For this review, take the finished solid that the model builds, in its own axes (mm). Face numbers are marked on the shaded views. A direction names the side the tool comes from. Give positions to 0.01 mm unless a question says otherwise; leave off trailing zeros. Order: outer loops, then holes, each group sorted by start corner. A loop starts at its lowest first (then second) coordinate and runs counter-clockwise, first axis right, second up. Notation, with made-up numbers: (37.5, -6.75) -> (62.5, -6.75) arc R18 cw to (62.5, 4.25) -> close; hole circle Ø10 at (4, 21.5). An arc over 180 degrees is marked (long way). Use CSV: the item, a comma, the result in double quotes. Start each with the question number.
Autodesk Inventor part; units mm, degrees
ref_plane "YZ Plane" through (0, 0, 0) normal (1, 0, 0) x (0, 1, 0)
ref_plane "XZ Plane" through (0, 0, 0) normal (0, 1, 0) x (-1, 0, 0)
ref_plane "XY Plane" through (0, 0, 0) normal (0, 0, 1) x (1, 0, 0)
sketch "스케치1" plane through (0, 0, 0) normal (0, 1, 0) x (-1, 0, 0)
  line L0 (4.1347, 105.7038) -> (-100.8653, 105.7038)
  line L1 (-100.8653, 105.7038) -> (-100.8653, -184.2962)
  line L2 (-100.8653, -184.2962) -> (4.1347, -184.2962)
  line L3 (4.1347, -184.2962) -> (4.1347, 105.7038)
  point P0 (0, 0)
  dimension "d0" = 105
  dimension "d1" = 290
sketch "스케치2" plane through (0, 0, 0) normal (0, 1, 0) x (-1, 0, 0)
  point P0 (0, 0)
sketch "스케치3" plane through (0, 0, 0) normal (0, 1, 0) x (-1, 0, 0)
  point P0 (0, 0)
sketch "스케치4" plane through (0, 0, 0) normal (0, 1, 0) x (-1, 0, 0)
  point P0 (0, 0)
extrude "돌출1" add sketch "스케치1" along normal blind 100
sketch "스케치5" plane through (100.8653, 0, 105.7038) normal (1, 0, 0) x (0, 0, -1)
  line L0 (0, 0) -> (290, 0)
  line L1 (290, 0) -> (285, 0)
  line L2 (285, 0) -> (285, 5)
  line L3 (285, 5) -> (290, 5)
  line L4 (290, 5) -> (290, 0)
  line L5 (290, 0) -> (290, 100)
  line L6 (290, 100) -> (285, 100)
  line L7 (285, 100) -> (285, 95)
  line L8 (285, 95) -> (290, 95)
  line L9 (290, 95) -> (290, 100)
  line L10 (285, 5) -> (35, 5)
  line L11 (35, 5) -> (35, 95)
  line L12 (35, 95) -> (285, 95)
  line L13 (285, 95) -> (285, 5)
  point P0 (105.7038, 0)
  dimension "d4" = 5
  dimension "d5" = 5
  dimension "d6" = 5
  dimension "d7" = 5
  dimension "d8" = 250
  dimension "d9" = 90
extrude "돌출2" cut sketch "스케치5" against normal blind 100 contours L10 L11 L12 L13
sketch "스케치6" plane through (100.8653, 0, 105.7038) normal (1, 0, 0) x (0, 0, -1)
  point P0 (105.7038, 0)
sketch "스케치7" plane through (100.8653, 0, 105.7038) normal (1, 0, 0) x (0, 0, -1)
  line L0 (285, 5) -> (35, 5)
  line L1 (35, 5) -> (11, 5)
  line L2 (11, 5) -> (11, 95)
  line L3 (11, 95) -> (35, 95)
  line L4 (35, 95) -> (35, 5)
  point P0 (105.7038, 0)
  dimension "d12" = 24
extrude "돌출3" cut sketch "스케치7" against normal blind 100
sketch "스케치8" plane through (-4.1347, 0, 105.7038) normal (0, 0, 1) x (1, 0, 0)
  circle A0 centre (22.6105, 17.0226) radius 10.2543
  point P0 (4.1347, 0)
sketch "스케치11" plane through (-4.1347, 0, -184.2962) normal (-1, 0, 0) x (0, 0, 1)
  point P0 (184.2962, 0)
sketch "스케치9" plane through (-4.1347, 0, -184.2962) normal (-1, 0, 0) x (0, 0, 1)
  line L0 (290, 100) -> (0, 100)
  line L1 (0, 100) -> (5, 100)
  line L2 (5, 100) -> (5, 95)
  line L3 (5, 95) -> (0, 95)
  line L4 (0, 95) -> (0, 100)
  line L5 (0, 0) -> (5, 0)
  line L6 (0, 0) -> (290, 0)
  line L7 (5, 0) -> (75, 0)
  line L8 (5, 0) -> (75, 0) construction
  line L9 (75, 0) -> (140, 0)
  line L10 (75, 0) -> (184.2962, 0)
  dimension "d15" = 5
  dimension "d16" = 5
  dimension "d17" = 5
  dimension "d18" = 70
  dimension "d19" = 0
  dimension "d20" = 65
sketch "스케치12" plane through (-4.1347, 0, -184.2962) normal (-1, 0, 0) x (0, 0, 1)
  point P0 (184.2962, 0)
sketch "스케치10" plane through (0, 0, 0) normal (0, -1, 0) x (1, 0, 0)
  point P0 (0, 0)
sketch "스케치13" plane through (-4.1347, 0, -184.2962) normal (-1, 0, 0) x (0, 0, 1)
  point P0 (184.2962, 0)
sketch "스케치14" plane through (0, 0, 0) normal (0, -1, 0) x (1, 0, 0)
  line L0 (-4.1347, -184.2962) -> (-4.1347, 105.7038)
  line L1 (-4.1347, -110.8863) -> (100.8653, -110.8863)
  line L2 (100.8653, 105.7038) -> (100.8653, -184.2962)
  line L3 (100.8653, -110.8863) -> (40.8653, -110.8863)
  line L4 (40.8653, -110.8863) -> (40.8653, -50.8863)
  line L5 (40.8653, -50.8863) -> (100.8653, -50.8863)
  line L6 (100.8653, -50.8863) -> (100.8653, -110.8863)
  point P0 (0, 0)
  dimension "d21" = 60
  dimension "d22" = 60
extrude "돌출4" cut sketch "스케치14" against normal blind 80
sketch "스케치15" plane through (0, 0, 0) normal (0, -1, 0) x (1, 0, 0)
  line L0 (100.8653, -184.2962) -> (-4.1347, -184.2962)
  line L1 (100.8653, -184.2962) -> (100.8653, -169.2962)
  line L2 (100.8653, -110.8863) -> (100.8653, -184.2962)
  line L3 (100.8653, -169.2962) -> (100.8653, -131.7962)
  circle A0 centre (100.8653, -131.7962) radius 37.5
  point P0 (0, 0)
  dimension "d25" = 15
  dimension "d26" = 37.5
  dimension "d27" = 75
extrude "돌출5" cut sketch "스케치15" against normal blind 80
sketch "스케치16" plane through (0, 0, 0) normal (0, -1, 0) x (1, 0, 0)
  arc A0 (69.7361, -110.8863) -> (100.8653, -169.2962) centre (100.8653, -131.7962) ccw
  line L0 (100.8653, -169.2962) -> (100.8653, -94.2962)
  line L1 (100.8653, 94.7038) -> (100.8653, -179.2962)
  line L2 (100.8653, -169.2962) -> (175.8653, -169.2962) construction
  line L3 (100.8653, -94.2962) -> (100.8653, -34.2962)
  line L4 (100.8653, -34.2962) -> (100.8653, 3.2038)
  circle A1 centre (100.8653, 3.2038) radius 37.5
  point P0 (0, 0)
  point P1 (100.8653, 40.7038)
  dimension "d30" = 75
  dimension "d31" = 90
  dimension "d32" = 60
  dimension "d33" = 37.5
  dimension "d34" = 180
  dimension "d35" = 75
extrude "돌출6" cut sketch "스케치16" against normal blind 8300 contours L1 A1 picked at (87.6481, -17.8312)
sketch "스케치17" plane through (0, 0, 0) normal (0, -1, 0) x (1, 0, 0)
  line L0 (100.8653, -34.2962) -> (100.8653, -184.2962)
  line L1 (100.8653, -184.2962) -> (100.8653, -169.0212)
  line L2 (100.8653, -169.0212) -> (100.8653, -131.5212)
  circle A0 centre (100.8653, -131.5212) radius 37.5
  point P0 (0, 0)
  point P1 (100.8653, -94.0212)
  dimension "d38" = 15.275
  dimension "d39" = 37.5
  dimension "d40" = 75
extrude "돌출7" cut sketch "스케치17" against normal blind 8300 contours L0 A0 picked at (87.6481, -152.5562)
sketch "스케치18" plane through (-4.1347, 0, -184.2962) normal (-1, 0, 0) x (0, 0, 1)
  line L0 (0, 0) -> (0, 100)
  line L1 (0, 50) -> (260, 50)
  line L2 (0, 50) -> (260, 50) construction
  point P0 (184.2962, 0)
  dimension "d43" = 260
  dimension "d44" = 0
sketch "스케치19" plane through (-4.1347, 0, -184.2962) normal (-1, 0, 0) x (0, 0, 1)
  line L0 (259.9404, 50.2138) -> (259.9404, 99.3471)
  line L1 (259.9404, 99.3471) -> (259.9404, 100)
  line L2 (290, 100) -> (225, 100)
  line L3 (290, 0) -> (225, 0)
  line L4 (259.9404, 100) -> (290, 100)
  line L5 (290, 100) -> (290, 0)
  line L6 (290, 0) -> (259.9404, 0)
  line L7 (259.9404, 0) -> (259.9404, 100)
  point P0 (184.2962, 0)
extrude "돌출8" cut sketch "스케치19" against normal blind 50
sketch "스케치24" plane through (100.8653, 0, -184.2962) normal (0, 0, -1) x (-1, 0, 0)
  line L0 (0, 0) -> (0, 5)
  line L1 (103, 100) -> (0, 100)
  line L2 (0, 100) -> (0, 0)
  line L3 (0, 0) -> (103, 0)
  line L4 (103, 0) -> (103, 100)
  point P0 (100.8653, 0)
extrude "돌출12" cut sketch "스케치24" against normal blind 3
sketch "스케치26" plane through (100.8653, 0, 105.7038) normal (0, 0, 1) x (1, 0, 0)
  line L0 (-55, 100) -> (0, 100)
  line L1 (0, 5) -> (0, 0)
  line L2 (-55, 100) -> (0, 100)
  line L3 (0, 100) -> (0, 0)
  line L4 (0, 0) -> (-55, 0)
  line L5 (-55, 0) -> (-55, 100)
  point P0 (-100.8653, 0)
extrude "돌출14" cut sketch "스케치26" against normal blind 7
fillet "모깎기7" radius 2 14 edges at (45.8653, 50, 98.7038) (73.3653, 100, 98.7038) (73.3653, 0, 98.7038) (45.8653, 50, 94.7038) (45.8653, 5, 85.1739) (23.3653, 5, 75.6441) (0.8653, 50, 75.6441) (-4.1347, 50, 75.6441) (23.3653, 95, 75.6441) (20.8653, 100, 75.6441) (20.8653, 0, 75.6441) (45.8653, 95, 85.1739) (45.8653, 100, 87.1739) (45.8653, 0, 87.1739)
sketch "스케치20" plane through (-4.1347, 98, -184.2962) normal (-1, 0, 0) x (0, 0, 1)
  line L0 (99.3624, -73.1284) -> (157.5725, -73.1284)
  line L1 (157.5725, -73.1284) -> (157.5725, -19.1517)
  line L2 (157.5725, -19.1517) -> (99.3624, -19.1517)
  line L3 (99.3624, -19.1517) -> (99.3624, -73.1284)
  point P0 (184.2962, -98)
sketch "스케치21" plane through (-14.1347, 98, -184.2962) normal (-1, 0, 0) x (0, 0, 1)
  line L0 (87.1912, -87.9455) -> (166.5686, -87.9455)
  line L1 (166.5686, -87.9455) -> (166.5686, -6.4514)
  line L2 (166.5686, -6.4514) -> (87.1912, -6.4514)
  line L3 (87.1912, -6.4514) -> (87.1912, -87.9455)
  line L4 (87.1912, -87.9455) -> (166.5686, -6.4514) construction
  line L5 (166.5686, -87.9455) -> (87.1912, -6.4514) construction
  point P0 (184.2962, -98)
  point P1 (126.8799, -47.1984)
sketch "스케치22" plane through (-24.1347, 98, -184.2962) normal (-1, 0, 0) x (0, 0, 1)
  line L0 (162.3351, -80.537) -> (95.6581, -80.537)
  line L1 (95.6581, -80.537) -> (95.6581, -12.8016)
  line L2 (95.6581, -12.8016) -> (162.3351, -12.8016)
  line L3 (162.3351, -12.8016) -> (162.3351, -80.537)
  line L4 (162.3351, -80.537) -> (95.6581, -12.8016) construction
  line L5 (95.6581, -80.537) -> (162.3351, -12.8016) construction
  point P0 (184.2962, -98)
  point P1 (128.9966, -46.6693)
properties part number "차체 뚜껑"
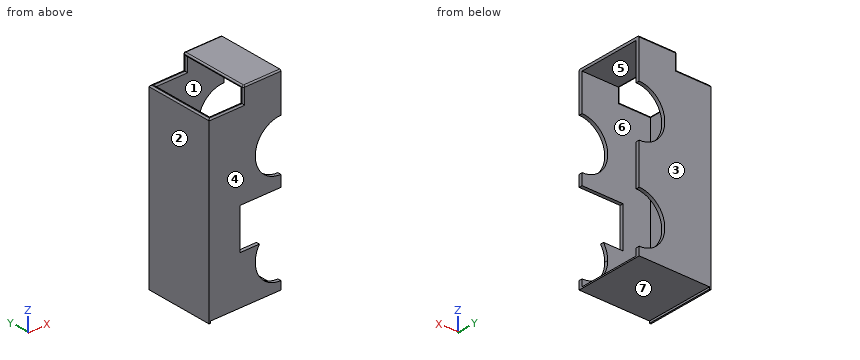
1. Draft analysis for pull direction Y (two halves, no side actions). For the marked faces 1, 2, 3 and 4, state which applies: +Y half, -Y half, draft (parallel to the pull), parting line (faces both ways), or undercut.
2. To check wall thickness, follow L1, parallel to Z at x = 72.5, y = 19; L2, parallel to Y at x = 23, z = 7; L3, parallel to Y at x = 61.5, z = -99. State the ranges of each line that lie inside material, in increasing order. Write a range as [from, to].
3. Consider section D-D (z = -147). State the section outline as (x, y) points, plus the area to 3 significant figures.
4. Consider section B-B (x = 17.5). State the section outline as (y, z) points, plus the area to 3 significant figures.
5. For the marked faces 5, 6 and 7, list the 3-axis set-ups (+Z, -Z, +X, -X, +Y, -Y) from which the entire face can be reached by the end or side of a thin tool; tool diameter is ignored.
6. Clearance check with flat-ended pins moving along their axes: P1, Ø5.5, axis at y = 3, z = -70, coming from the +X side; P2, Ø1.5, axis at x = 69, y = 3.5, coming from the -Z side; P3, Ø2.5, axis at y = 51, z = -182.5, coming from the +X side; P4, Ø1.5, axis at y = 78, z = -137.5, coming from the +X side. State where each tip first meets the part, or that it passes through.
7. Consider section C-C (z = -62). State the section outline as (x, y) points.
Answer list:
1,face 1,"undercut"
1,face 2,"draft"
1,face 3,"+Y half"
1,face 4,"-Y half"
2,L1,"[-181.3, -179.3], [94.7, 98.7]"
2,L2,"[0, 5], [95, 100]"
2,L3,"[95, 100]"
3,outline,"(-4.13, 0) -> (66.59, 0) -> (66.59, 5) -> (0.87, 5) -> (0.87, 95) -> (66.71, 95) -> (66.71, 100) -> (-4.13, 100) -> close"
3,area,"1,160 mm2"
4,outline,"(0, -181.3) -> (100, -181.3) -> (100, 73.64) arc R2 ccw to (98, 75.64) -> (97, 75.64) arc R2 ccw to (95, 73.64) -> (95, -179.3) -> (5, -179.3) -> (5, 73.64) arc R2 ccw to (3, 75.64) -> (2, 75.64) arc R2 ccw to (0, 73.64) -> close"
4,area,"2,750 mm2"
5,face 5,"+X, -X"
5,face 6,"+X"
5,face 7,"-Z, +X, +Y, -Y"
6,P1,"x = 40.87"
6,P2,"z = -181.3"
6,P3,"x = 100.87"
6,P4,"x = 0.87"
7,outline,"(-4.13, 0) -> (40.87, 0) -> (40.87, 5) -> (0.87, 5) -> (0.87, 95) -> (100.87, 95) -> (100.87, 100) -> (-4.13, 100) -> close"
